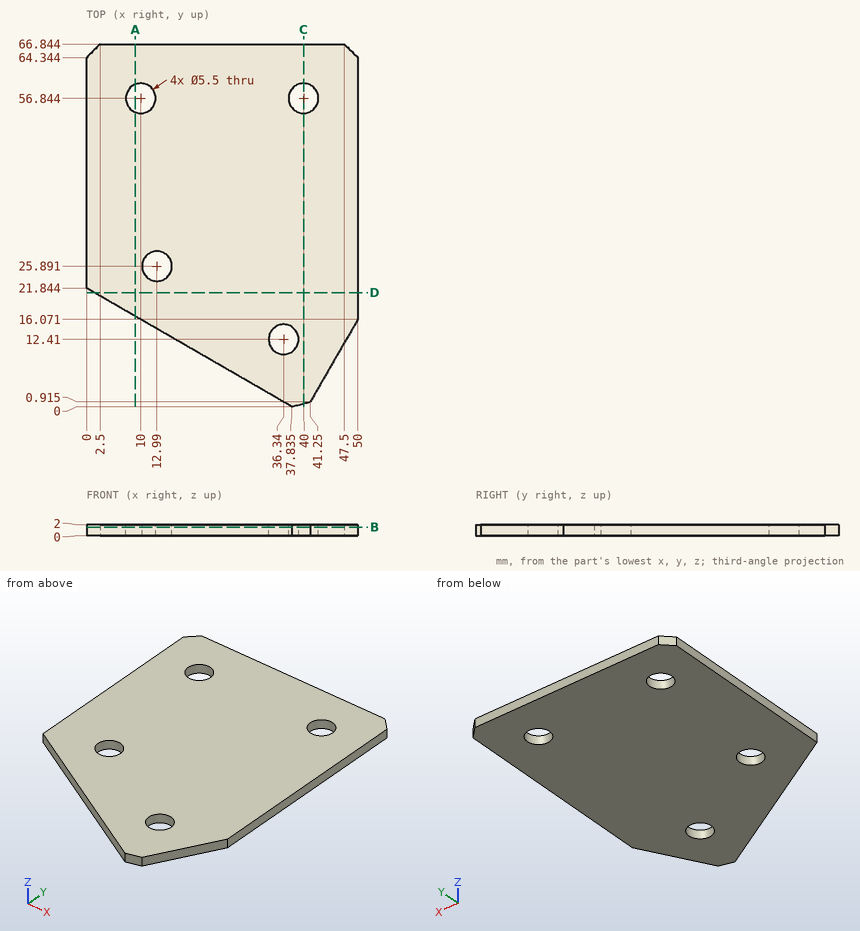
Design review of the part shown in the three views and the two pictorial views. Dimensions are in mm from the part's minimum x, y and z. Round coordinates to 2 decimals unless told otherwise and drop trailing zeros. Loops run counter-clockwise (first coordinate to the right, second up) from the corner with the lowest first, then second, coordinate; pieces in that order, holes last. Notation, with made-up numbers: M 45,-0.5 L 93,-0.5 A23 ccw 93,23.5 Z; hole C 31,-17 d5. An arc over 180 degrees is marked long. Answer as a JSON object with one key per item and string values.
Item 1: We need section A-A on x = 9. Give the boundary of the cut face in (y, z) (1 decimal).
Answer sheet:
{"outline": "M 16.6,0 L 54.3,0 L 54.3,2 L 16.6,2 Z; M 59.4,0 L 66.8,0 L 66.8,2 L 59.4,2 Z"}
Item 2: We need section C-C on x = 40. Give the boundary of the cut face in (y, z) (1 decimal).
Answer sheet:
{"outline": "M 0.6,0 L 54.1,0 L 54.1,2 L 0.6,2 Z; M 59.6,0 L 66.8,0 L 66.8,2 L 59.6,2 Z"}
Item 3: We need section B-B on z = 1.55. State how many separate pieces and enclosed holes the cut face has, and give its area (3 significant figures).
Answer sheet:
{"separate pieces": "1", "enclosed holes": "4", "area": "2,750 mm^2"}
Item 4: We need section D-D on y = 21. Give the boundary of the cut face in (x, z).
Answer sheet:
{"outline": "M 1.46,0 L 50,0 L 50,2 L 1.46,2 Z"}
Item 5: Clearance check with flat-ended pins moving along their axes: P1, Ø3.5, axis at x = 40, y = 56.84, coming from the +Z side; P2, Ø1, axis at y = 11, z = 0.5, coming from the +X side. State where each tip first meets the part, or that it passes through.
Answer sheet:
{"P1": "passes through", "P2": "stops at x = 47.36"}
Item 6: Wall thickness on L1, parallel to X at y = 55.5, z = 0.4; L2, parallel to Y at x = 40, z = 1.35 (1 decimal); L3, parallel to X at y = 56, z = 0.15: over which ranges is each line inside the solid? List them lowest first. Write a range as from..to.
Answer sheet:
{"L1": "x = 0..7.6, 12.4..37.6, 42.4..50", "L2": "y = 0.6..54.1, 59.6..66.8", "L3": "x = 0..7.38, 12.62..37.38, 42.62..50"}
